```python
from build123d import *

# Parameters (mm, degrees)
F0_R     = 7.5
F1_DEPTH = 20
F2_R     = 5
F3_DEPTH = 15
F4_W     = 3.4
F4_H     = 3.4
F5_DEPTH = 10


with BuildPart() as f1:
    # F0 (on Top) → F1 (new body)
    with BuildSketch(Plane.XY):
        Circle(F0_R)
    extrude(amount=F1_DEPTH)

    # F2 (on face) → F3 (cut)
    with BuildSketch(Plane.XY.offset(20)):
        Circle(F2_R)
    extrude(amount=-F3_DEPTH, mode=Mode.SUBTRACT)

    # F4 (on face) → F5 (cut)
    with BuildSketch(Plane(origin=(0, 0, 0), x_dir=(1, 0, 0), z_dir=(0, 0, -1))):
        Rectangle(F4_W, F4_H)
    extrude(amount=-F5_DEPTH, mode=Mode.SUBTRACT)


solid = f1.part
```
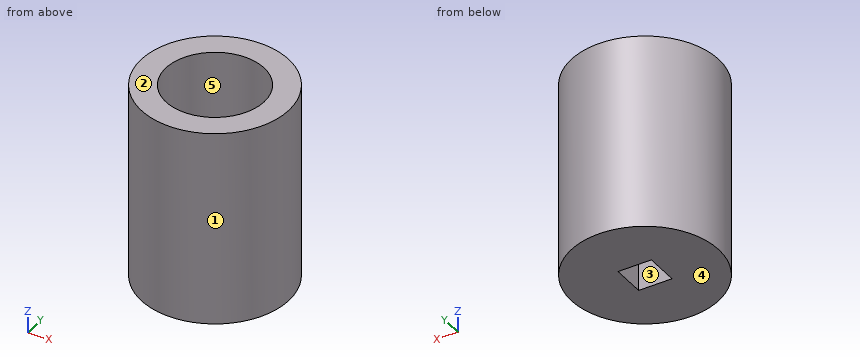
Here's how the part is built. I have some questions about the finished solid (model axes, mm). Face numbers are marked on the shaded views. A direction names the side the tool comes from. Coordinates: 2 decimals unless noted, no trailing zeros. Order: outer loops, then holes, each group sorted by start corner. A loop starts at its lowest first (then second) coordinate and runs counter-clockwise, first axis right, second up.
1) Will these pins go through, and if not, where does the flat tip stop? pin 1 (6 mm diameter, centred on x = 0, y = 0, fed in from +Z); pin 2 (1.5 mm diameter, centred on x = -5.5, z = 16, fed in from -Y); pin 3 (8 mm diameter, centred on y = 5.5, z = 7, fed in from +X).
2) Imagine slicing it at A-A on y = 0. List the corners of the cut face in (x, z) for me, and give its area (3 significant figures).
3) Imagine slicing it at D-D on x = 4.75. List the corners of the cut face in (y, z) for me.
4) Imagine slicing it at C-C on z = 4.75. List the corners of the cut face in (x, y) for me.
5) Which directions (+Z, -Z, +X, -X, +Y, -Y) give clear straight access to the entire face, cutting with the end or side of a thin tool? Please do the marked faces 4 and 5.
6) I need wall thicknesses on line 1 (Y direction, x = 0, z = 13.75); line 2 (Z direction, x = 0.5, y = -3.25); line 3 (X direction, y = -3.25, z = 9). Which ranges of each line are inside material? Lowest first, please.
7) We'd pull the mould along Y, two halves only. Please class the marked faces 1, 2 and 3: +Y half, -Y half, draft (parallel to the pull), parting line (faces both ways), or undercut.
Response values:
1. pin 1: stops at z = 5
1. pin 2: stops at y = -5.8
1. pin 3: stops at x = 7.35
2. outline: (-7.5, 0) - (-1.7, 0) - (-1.7, 5) - (-5, 5) - (-5, 20) - (-7.5, 20) - close; (1.7, 0) - (7.5, 0) - (7.5, 20) - (5, 20) - (5, 5) - (1.7, 5) - close
2. area: 133 mm2
3. outline: (-5.8, 0) - (5.8, 0) - (5.8, 20) - (1.56, 20) - (1.56, 5) - (-1.56, 5) - (-1.56, 20) - (-5.8, 20) - close
4. outline: circle Ø15 at (0, 0); hole (-1.7, -1.7) - (1.7, -1.7) - (1.7, 1.7) - (-1.7, 1.7) - close
5. face 4: -Z, +X, -X, +Y, -Y
5. face 5: +Z
6. line 1: y = -7.5 to -5, 5 to 7.5
6. line 2: z = 0 to 5
6. line 3: x = -6.76 to -3.8, 3.8 to 6.76
7. face 1: parting line
7. face 2: draft
7. face 3: undercut
